```python
from build123d import *

# Parameters (mm, degrees)
SKETCH1_W                 = 101.6
SKETCH1_H                 = 53.34
BOSS_EXTRUDE1_DEPTH       = 4.7625
FILLET1_R                 = 2.54
TAP_DRILL_FOR_4_40_TAP1_D = 2.2606
F_4_CLEARANCE_HOLE2_D     = 2.9464


with BuildPart() as part:
    # Sketch1 → Boss-Extrude1 (new body)
    with BuildSketch(Plane.XY):
        with Locations((50.8, 26.67)):
            Rectangle(SKETCH1_W, SKETCH1_H)
    extrude(amount=BOSS_EXTRUDE1_DEPTH)

    # Fillet1
    fillet1_edges = [part.edges().sort_by_distance(p)[0] for p in [
        (0, 53.34, 2.38125),
        (101.6, 53.34, 2.38125),
        (101.6, 0, 2.38125),
        (0, 0, 2.38125),
    ]]
    fillet(fillet1_edges, radius=FILLET1_R)

    # Tap Drill for #4-40 Tap1 (through all)
    with Locations(Plane(origin=(0, 0, 0), x_dir=(-1, 0, 0), z_dir=(0, 0, -1))):
        with Locations((-15.24, 2.54), (-90.17, 2.54), (-96.52, 50.8), (-66.04, 17.78), (-66.04, 45.72), (-13.97, 50.8)):
            Hole(TAP_DRILL_FOR_4_40_TAP1_D / 2)

    # #4 Clearance Hole2 (through all)
    with Locations(Plane.XY.offset(4.7625)):
        with Locations((9.525, 42.418), (9.525, 10.668), (92.075, 42.418), (92.075, 10.668)):
            Hole(F_4_CLEARANCE_HOLE2_D / 2)


solid = part.part
```
The model under review builds one solid part; all positions refer to its coordinate system, in mm. Round coordinates to 2 decimals unless told otherwise and drop trailing zeros. Order: outer loops, then holes, each group sorted by start corner. A loop starts at its lowest first (then second) coordinate and runs counter-clockwise, first axis right, second up. Notation, with made-up numbers: M -22,47 L 24,47 A29 ccw 24,76 Z; hole C 5.5,-27 d6. An arc over 180 degrees is marked long. Use a Markdown table: item, result.
1) Insertion check: pin 1 (1.8 mm diameter, centred on x = 96.52, y = 50.8, fed in from +Z). The pin has a flat end and moves straight along its axis. Give the tip position at first contact, or say it passes through.
Report:
| item | result |
|---|---|
| pin 1 | through |
2) Draft analysis for pull direction X (two halves, no side actions). For faces 1 (the face through (9.72, 43.88, 2.35)), 2 (the face through (101.6, 26, 2)), 3 (the face through (50, 27, 4.762)), state which applies: released by +X, released by -X, zero draft, split by the parting line, or undercut.
Report:
| item | result |
|---|---|
| face 1 | undercut |
| face 2 | released by +X |
| face 3 | zero draft |
3) Consider section A-A (y = 17.78). Write out the cut boundary in (x, z), then the cut area to 3 significant figures.
Report:
| item | result |
|---|---|
| outline | M 0,0 L 64.91,0 L 64.91,4.76 L 0,4.76 Z; M 67.17,0 L 101.6,0 L 101.6,4.76 L 67.17,4.76 Z |
| area | 473 mm^2 |
4) Consider section B-B (x = 66.04). Write out the cut boundary in (y, z), then the cut area to 4 significant figures.
Report:
| item | result |
|---|---|
| outline | M 0,0 L 16.65,0 L 16.65,4.76 L 0,4.76 Z; M 18.91,0 L 44.59,0 L 44.59,4.76 L 18.91,4.76 Z; M 46.85,0 L 53.34,0 L 53.34,4.76 L 46.85,4.76 Z |
| area | 232.5 mm^2 |
5) Wall thickness on line 1 along Y through (x, z) = (92, 2.7); line 2 along Y through (x, z) = (66.04, 2); line 3 along X through (y, z) = (2, 3.5): over which ranges is each line inside the solid? List them lowest first. Write a range as [from, to].
Report:
| item | result |
|---|---|
| line 1 | [0, 9.2], [12.14, 40.95], [43.89, 53.34] |
| line 2 | [0, 16.65], [18.91, 44.59], [46.85, 53.34] |
| line 3 | [0.06, 14.25], [16.23, 89.18], [91.16, 101.54] |
